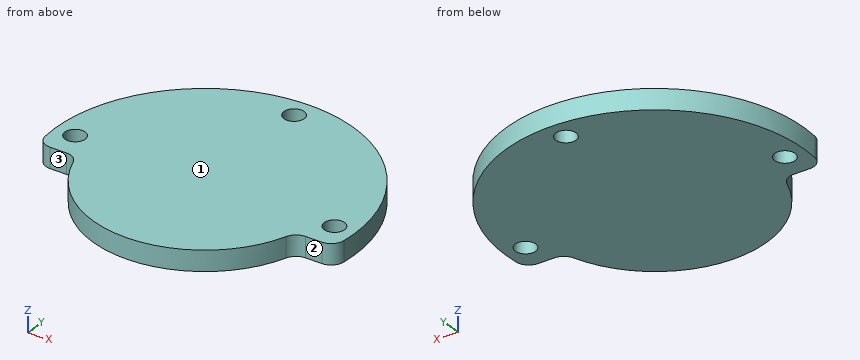
from build123d import *

# Parameters (mm, degrees)
SKETCH_1_R      = 1.5
EXTRUDE_1_DEPTH = 3
FILLET_1_R      = 2


with BuildPart() as part:
    # 草图1 → 凸台-拉伸1 (new body)
    with BuildSketch(Plane.XY):
        with BuildLine():
            Line((-16.007810594, -4), (-21.633307653, -4))
            ThreePointArc((-21.633307653, -4), (0, 22), (21.633307653, -4))
            Line((21.633307653, -4), (16.007810594, -4))
            ThreePointArc((16.007810594, -4), (0, -16.5), (-16.007810594, -4))
        make_face()
        with Locations((-19, 0)):
            Circle(SKETCH_1_R, mode=Mode.SUBTRACT)
        with Locations((0, 19)):
            Circle(SKETCH_1_R, mode=Mode.SUBTRACT)
        with Locations((19, 0)):
            Circle(SKETCH_1_R, mode=Mode.SUBTRACT)
    extrude(amount=EXTRUDE_1_DEPTH)

    # 圆角1
    fillet_1_edges = [part.edges().sort_by_distance(p)[0] for p in [
        (-16.007810594, -4, 1.5),
        (-21.633307653, -4, 1.5),
        (21.633307653, -4, 1.5),
        (16.007810594, -4, 1.5),
    ]]
    fillet(fillet_1_edges, radius=FILLET_1_R)


solid = part.part
Geometry: final body of the model. Coordinates: model frame, mm. Face numbers are marked on the shaded views. A direction names the side the tool comes from. Coordinates: 2 decimals unless noted, no trailing zeros. Order: outer loops, then holes, each group sorted by start corner. A loop starts at its lowest first (then second) coordinate and runs counter-clockwise, first axis right, second up.
1) Section A-A (x = 0). Return loops of the section in (y, z).
Result sheet:
outline: (-16.5, 0) - (17.5, 0) - (17.5, 3) - (-16.5, 3) - close; (20.5, 0) - (22, 0) - (22, 3) - (20.5, 3) - close
2) Ray query, probe 1 along X at (y, z) = (-0.5, 1.35); probe 2 along Y at (x, z) = (19, 1); probe 3 along X at (y, z) = (18, 1). Return the intervals inside material, ascending.
Result sheet:
probe 1: x = -21.99 to -20.41, -17.59 to 17.59, 20.41 to 21.99
probe 2: y = -4 to -1.5, 1.5 to 11.09
probe 3: x = -12.65 to -1.12, 1.12 to 12.65
3) Set-up query: the marked faces 1, 2 and 3. Return all of +Z, -Z, +X, -X, +Y, -Y with unobstructed straight access to the full face (end or side cutting, diameter ignored); none if empty.
Result sheet:
face 1: +Z, +X, -X, +Y, -Y
face 2: +Z, -Z, +X, -Y
face 3: +Z, -Z, -X, -Y
4) Section C-C (z = 2.1). Return loops of the section in (x, y), then the cut area to 3 significant figures.
Result sheet:
outline: (-21.89, -2.2) arc R2 ccw to (-19.9, -4) - (-17.5, -4) arc R2 cw to (-15.61, -5.35) arc R16.5 ccw to (15.61, -5.35) arc R2 cw to (17.5, -4) - (19.9, -4) arc R2 ccw to (21.89, -2.2) arc R22 ccw (long way) to start; hole circle Ø3 at (-19, 0); hole circle Ø3 at (0, 19); hole circle Ø3 at (19, 0)
area: 1,210 mm2
5) Section D-D (y = 19). Return loops of the section in (x, z), then the cut area to 3 significant figures.
Result sheet:
outline: (-11.09, 0) - (-1.5, 0) - (-1.5, 3) - (-11.09, 3) - close; (1.5, 0) - (11.09, 0) - (11.09, 3) - (1.5, 3) - close
area: 57.5 mm2
6) Section B-B (y = 0). Return loops of the section in (x, z), then the cut area to 3 significant figures.
Result sheet:
outline: (-22, 0) - (-20.5, 0) - (-20.5, 3) - (-22, 3) - close; (-17.5, 0) - (17.5, 0) - (17.5, 3) - (-17.5, 3) - close; (20.5, 0) - (22, 0) - (22, 3) - (20.5, 3) - close
area: 114 mm2
7) First-contact query: P1, Ø5, axis at x = 19, y = 0, coming from the +Z side. Flat tip, straight axial feed; report the tip coordinate or a pass-through.
Result sheet:
P1: stops at z = 3
